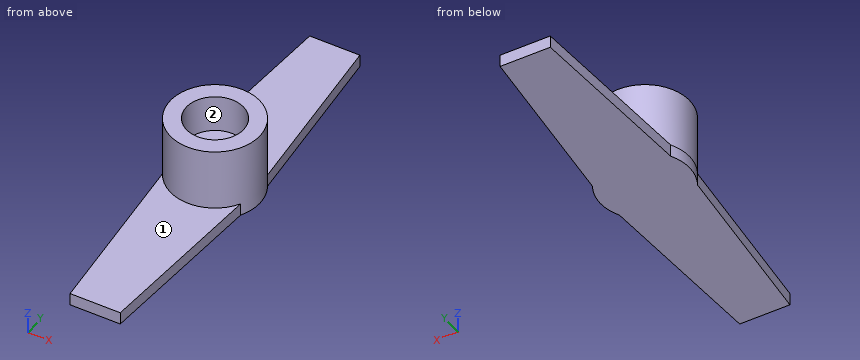
from build123d import *

# Parameters (mm, degrees)
SALIENTE_EXTRUIR1_DEPTH = 1
CROQUIS2_R              = 3.6
SALIENTE_EXTRUIR2_DEPTH = 5
CROQUIS3_R              = 2.3
CORTAR_EXTRUIR1_DEPTH   = 3


with BuildPart() as part:
    # Croquis1 → Saliente-Extruir1 (new body)
    with BuildSketch(Plane.XY):
        with BuildLine():
            Line((-2, -16), (2, -16))
            Line((2, -16), (3.117691454, -1.8))
            ThreePointArc((3.117691454, -1.8), (3.6, 0), (3.117691454, 1.8))
            Line((3.117691454, 1.8), (2, 16))
            Line((2, 16), (-2, 16))
            Line((-2, 16), (-3.117691454, 1.8))
            ThreePointArc((-3.117691454, 1.8), (-3.6, 0), (-3.117691454, -1.8))
            Line((-3.117691454, -1.8), (-2, -16))
        make_face()
    extrude(amount=SALIENTE_EXTRUIR1_DEPTH)

    # Croquis2 → Saliente-Extruir2 (add)
    with BuildSketch(Plane.XY.offset(1)):
        Circle(CROQUIS2_R)
    extrude(amount=SALIENTE_EXTRUIR2_DEPTH)

    # Croquis3 → Cortar-Extruir1 (cut)
    with BuildSketch(Plane.XY.offset(6)):
        Circle(CROQUIS3_R)
    extrude(amount=-CORTAR_EXTRUIR1_DEPTH, mode=Mode.SUBTRACT)


solid = part.part
Design review of the part built by this model. Coordinates are the model's own, in mm. Face numbers are marked on the shaded views. Round coordinates to 2 decimals unless told otherwise and drop trailing zeros. Loops run counter-clockwise (first coordinate to the right, second up) from the corner with the lowest first, then second, coordinate; pieces in that order, holes last. Notation, with made-up numbers: (-29, -22) - (-2, -22) arc R15 ccw to (-2, 3) - close; hole circle Ø11 at (49, 4.25). An arc over 180 degrees is marked (long way). One line per question, with ' | ' between items.
1. Clearance check with flat-ended pins moving along their axes: P1, Ø4, axis at x = 0, y = -11.5, coming from the +Z side; P2, Ø2, axis at x = 0, z = 5.5, coming from the -Y side. State where each tip first meets the part, or that it passes through.
Results are:
P1: stops at z = 1 | P2: stops at y = -3.6
2. Draft analysis for pull direction X (two halves, no side actions). For the marked faces 1 and 2, state which applies: released by +X, released by -X, zero draft, split by the parting line, or undercut.
Results are:
face 1: zero draft | face 2: undercut
3. We need section C-C, the plane y = 1.5. State the section outline as (x, z) points, and give its area (3 significant figures).
Results are:
outline: (-3.27, 0) - (3.27, 0) - (3.27, 6) - (1.74, 6) - (1.74, 3) - (-1.74, 3) - (-1.74, 6) - (-3.27, 6) - close | area: 28.8 mm²
4. We need section A-A, the plane x = 0. State the section outline as (y, z) points.
Results are:
outline: (-16, 0) - (16, 0) - (16, 1) - (3.6, 1) - (3.6, 6) - (2.3, 6) - (2.3, 3) - (-2.3, 3) - (-2.3, 6) - (-3.6, 6) - (-3.6, 1) - (-16, 1) - close
5. We need section B-B, the plane z = 4.9. State the section outline as (x, y) points, and give its area (3 significant figures).
Results are:
outline: circle Ø7.2 at (0, 0); hole circle Ø4.6 at (0, 0) | area: 24.1 mm²
6. We need section D-D, the plane x = 2.75. State the section outline as (y, z) points, and give its area (3 significant figures).
Results are:
outline: (-6.47, 0) - (6.47, 0) - (6.47, 1) - (2.32, 1) - (2.32, 6) - (-2.32, 6) - (-2.32, 1) - (-6.47, 1) - close | area: 36.2 mm²
7. For L1, parallel to Y at x = 0, z = 4.4; L2, parallel to Z at x = 1, y = -12; L3, parallel to Y at x = -0.5, z = 4.85 (3 decimals), list the stretches that pass through material, from the lowest coordinate up. Write a range as [from, to].
Results are:
L1: y = [-3.6, -2.3], [2.3, 3.6] | L2: z = [0, 1] | L3: y = [-3.565, -2.245], [2.245, 3.565]
